Could you check a few things on this drawing? It's one solid part, dimensions in mm from its lowest x, y, z. A direction names the side the tool comes from. Give positions to 0.01 mm unless a question says otherwise; leave off trailing zeros. Loops run counter-clockwise (first coordinate to the right, second up) from the corner with the lowest first, then second, coordinate; pieces in that order, holes last. Notation, with made-up numbers: (-39, 10.5) - (4, 10.5) arc R18 cw to (4, 21.5) - close; hole circle Ø1 at (17.25, 7). An arc over 180 degrees is marked (long way). Return JSON: item names as keys, results as strings. Group by question number.
(1) If we section it at B-B (z = 11.5): Please give me the cut outline in (x, y) (1 decimal), then the cut area to 3 significant figures.
(2) If we mould it in two halves opening along Y, with no side actions, what happens to the marked faces 4, 5 and 6? For each: released by +Y, released by -Y, zero draft, split by the parting line, or undercut.
(3) For P1, Ø8, axis at y = 46.5, z = 29, coming from the +X side; P2, Ø5.5, axis at y = 29, z = 11.5, coming from the +X side, each with a flat end and sliding along its axis, tell me the tip position at first contact or that it passes through.
(4) If we section it at C-C (y = 58): Please give me the cut outline in (x, z), then the cut area to 3 significant figures.
(5) On a 3-axis mill with a long thin cutter (end or side, diameter ignored), from which of +Z, -Z, +X, -X, +Y, -Y can I reach the whole of each face in a straight line? I mean the marked faces 1, 2 and 3. Say none if no direction works.
(6) I need wall thicknesses on probe 1 along Y at (x, z) = (87, 9) (1 decimal); probe 2 along X at (y, z) = (37, 48); probe 3 along X at (y, z) = (22, 3). Which ranges of each line are inside material? Lowest first, please. Write a range as [from, to].
(7) If we section it at D-D (x = 63): Please give me the cut outline in (y, z).
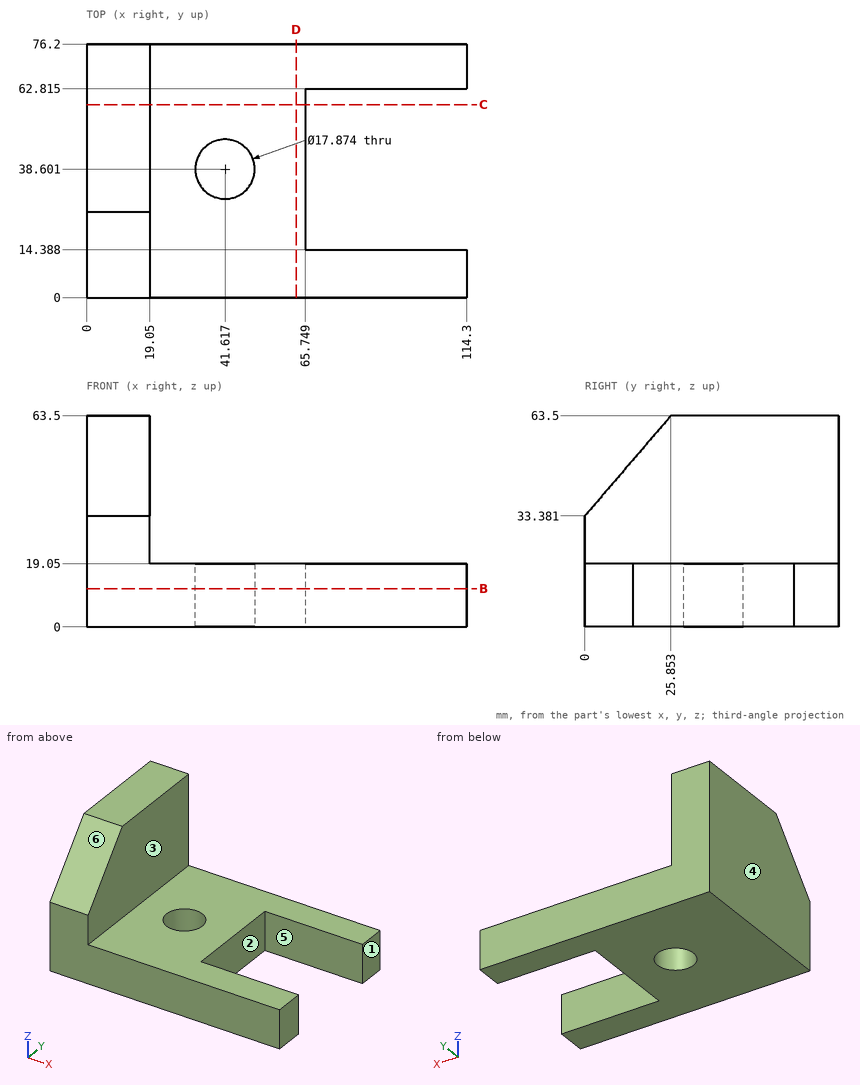
Values:
{
 "1": {"outline": "(0, 0) - (114.3, 0) - (114.3, 14.4) - (65.7, 14.4) - (65.7, 62.8) - (114.3, 62.8) - (114.3, 76.2) - (0, 76.2) - close; hole circle Ø17.9 at (41.6, 38.6)", "area": "6,110 mm2"},
 "2": {"face 4": "zero draft", "face 5": "undercut", "face 6": "released by -Y"},
 "3": {"P1": "x = 19.05", "P2": "x = 65.75"},
 "4": {"outline": "(0, 0) - (65.75, 0) - (65.75, 19.05) - (19.05, 19.05) - (19.05, 63.5) - (0, 63.5) - close", "area": "2,100 mm2"},
 "5": {"face 1": "+Z, -Z, +X, +Y, -Y", "face 2": "+Z, -Z, +X", "face 3": "+Z, +X, +Y, -Y"},
 "6": {"probe 1": "[0, 14.4], [62.8, 76.2]", "probe 2": "[0, 19.05]", "probe 3": "[0, 65.75]"},
 "7": {"outline": "(0, 0) - (76.2, 0) - (76.2, 19.05) - (0, 19.05) - close"}
}
